from build123d import *

# Parameters (mm, degrees)
SKETCH1_R           = 27.5
SKETCH1_R_2         = 5
BOSS_EXTRUDE1_DEPTH = 25
CUT_EXTRUDE1_DEPTH  = 25
SKETCH3_R           = 30
SKETCH3_R_2         = 27.25
BOSS_EXTRUDE2_DEPTH = 25


with BuildPart() as part:
    # Sketch1 → Boss-Extrude1 (new body)
    with BuildSketch(Plane(origin=(0, 0, 0), x_dir=(0, 0, -1), z_dir=(1, 0, 0))):
        Circle(SKETCH1_R)
        Circle(SKETCH1_R_2, mode=Mode.SUBTRACT)
    extrude(amount=BOSS_EXTRUDE1_DEPTH)

    # Sketch2 → Cut-Extrude1 (cut)
    with BuildSketch(Plane(origin=(25, 0, 0), x_dir=(0, 0, -1), z_dir=(1, 0, 0))):
        with BuildLine():
            Line((-2.5, 27.386127875), (-2.5, 9.386127875))
            ThreePointArc((-2.5, 9.386127875), (-3.356749875, 8.103911075), (-4.869227717, 8.404761623))
            Line((-4.869227717, 8.404761623), (-17.597149778, 21.132683684))
            ThreePointArc((-17.597149778, 21.132683684), (-10.670518583, 25.760910681), (-2.5, 27.386127875))
        make_face()
        with BuildLine():
            Line((17.597149778, 21.132683684), (4.869227717, 8.404761623))
            ThreePointArc((4.869227717, 8.404761623), (3.356749875, 8.103911075), (2.5, 9.386127875))
            Line((2.5, 9.386127875), (2.5, 27.386127875))
            ThreePointArc((2.5, 27.386127875), (10.670518583, 25.760910681), (17.597149778, 21.132683684))
        make_face()
        with BuildLine():
            Line((27.386127875, 2.5), (9.386127875, 2.5))
            ThreePointArc((9.386127875, 2.5), (8.103911075, 3.356749875), (8.404761623, 4.869227717))
            Line((8.404761623, 4.869227717), (21.132683684, 17.597149778))
            ThreePointArc((21.132683684, 17.597149778), (25.760910681, 10.670518583), (27.386127875, 2.5))
        make_face()
        with BuildLine():
            Line((21.132683684, -17.597149778), (8.404761623, -4.869227717))
            ThreePointArc((8.404761623, -4.869227717), (8.103911075, -3.356749875), (9.386127875, -2.5))
            Line((9.386127875, -2.5), (27.386127875, -2.5))
            ThreePointArc((27.386127875, -2.5), (25.760910681, -10.670518583), (21.132683684, -17.597149778))
        make_face()
        with BuildLine():
            Line((2.5, -27.386127875), (2.5, -9.386127875))
            ThreePointArc((2.5, -9.386127875), (3.356749875, -8.103911075), (4.869227717, -8.404761623))
            Line((4.869227717, -8.404761623), (17.597149778, -21.132683684))
            ThreePointArc((17.597149778, -21.132683684), (10.670518583, -25.760910681), (2.5, -27.386127875))
        make_face()
        with BuildLine():
            Line((-17.597149778, -21.132683684), (-4.869227717, -8.404761623))
            ThreePointArc((-4.869227717, -8.404761623), (-3.356749875, -8.103911075), (-2.5, -9.386127875))
            Line((-2.5, -9.386127875), (-2.5, -27.386127875))
            ThreePointArc((-2.5, -27.386127875), (-10.670518583, -25.760910681), (-17.597149778, -21.132683684))
        make_face()
        with BuildLine():
            Line((-27.386127875, -2.5), (-9.386127875, -2.5))
            ThreePointArc((-9.386127875, -2.5), (-8.103911075, -3.356749875), (-8.404761623, -4.869227717))
            Line((-8.404761623, -4.869227717), (-21.132683684, -17.597149778))
            ThreePointArc((-21.132683684, -17.597149778), (-25.760910681, -10.670518583), (-27.386127875, -2.5))
        make_face()
        with BuildLine():
            Line((-21.132683684, 17.597149778), (-8.404761623, 4.869227717))
            ThreePointArc((-8.404761623, 4.869227717), (-8.103911075, 3.356749875), (-9.386127875, 2.5))
            Line((-9.386127875, 2.5), (-27.386127875, 2.5))
            ThreePointArc((-27.386127875, 2.5), (-25.760910681, 10.670518583), (-21.132683684, 17.597149778))
        make_face()
    extrude(amount=-CUT_EXTRUDE1_DEPTH, mode=Mode.SUBTRACT)

    # Sketch3 → Boss-Extrude2 (add)
    with BuildSketch(Plane(origin=(25, 0, 0), x_dir=(0, 0, -1), z_dir=(1, 0, 0))):
        Circle(SKETCH3_R)
        Circle(SKETCH3_R_2, mode=Mode.SUBTRACT)
    extrude(amount=-BOSS_EXTRUDE2_DEPTH)


solid = part.part
Source: CAD feature listing. Evaluate the final solid. Frame: model axes, mm. Coordinates: 2 decimals unless noted, no trailing zeros. Order: outer loops, then holes, each group sorted by start corner. A loop starts at its lowest first (then second) coordinate and runs counter-clockwise, first axis right, second up. Notation, with made-up numbers: M -17.75,72 L -8.75,72 A19 cw -8.75,86 Z; hole C 58.25,73 d8. An arc over 180 degrees is marked long. Write each question's results on one line, items separated by ' | '. Start each with the question number.
Item 1: Draft query along Y for faces 1 (the face through (0, 0, -6)), 2 (the face through (12.68, 1.32, 29.97)), 3 (the face through (12.675, 11.232, 14.768)). Return one class per face: pulls with the +Y half, pulls with the -Y half, needs draft (parallel to the pull), parting line crosses it, or undercut.
Item 2: Line query: probe 1 along Y at (x, z) = (12.5, 0); probe 2 along Z at (x, y) = (17.75, -22.5); probe 3 along Z at (x, y) = (4, -24.5). Output: solid intervals per line, ascending.
Item 3: Cut plane C-C (x = 2.5). Count the separate pieces of the cut face and the enclosed holes in it, and give its area (3 significant figures).
Item 4: First-contact query: pin 1 Ø6 at (x, z) = (12, 22) entering from -Y; pin 2 Ø4 at (x, z) = (10.5, 8) entering from +Y; pin 3 Ø9 at (x, z) = (12.5, -21.5) entering from +Y. Flat tips, straight axial feed; report the tip coordinate or a pass-through.
Item 5: Cut plane D-D (z = 23.5). Return loops of the section in (x, y).
Item 6: Cut plane A-A (z = 0). Return loops of the section in (x, y).
Checked values:
1) face 1: needs draft | face 2: parting line crosses it | face 3: undercut
2) probe 1: y = -30 to -5, 5 to 30 | probe 2: z = -19.84 to -15.37, -2.5 to 2.5, 15.37 to 19.84 | probe 3: z = -17.31 to -11.93, -2.5 to 2.5, 11.93 to 17.31
3) separate pieces: 1 | enclosed holes: 9 | area: 1,400 mm2
4) pin 1: stops at y = -23.22 | pin 2: stops at y = 29.39 | pin 3: stops at y = 24.72
5) outline: M 0,-18.65 L 25,-18.65 L 25,-13.8 L 0,-13.8 Z; M 0,-2.5 L 25,-2.5 L 25,2.5 L 0,2.5 Z; M 0,13.8 L 25,13.8 L 25,18.65 L 0,18.65 Z
6) outline: M 0,-30 L 25,-30 L 25,-5 L 0,-5 Z; M 0,5 L 25,5 L 25,30 L 0,30 Z
